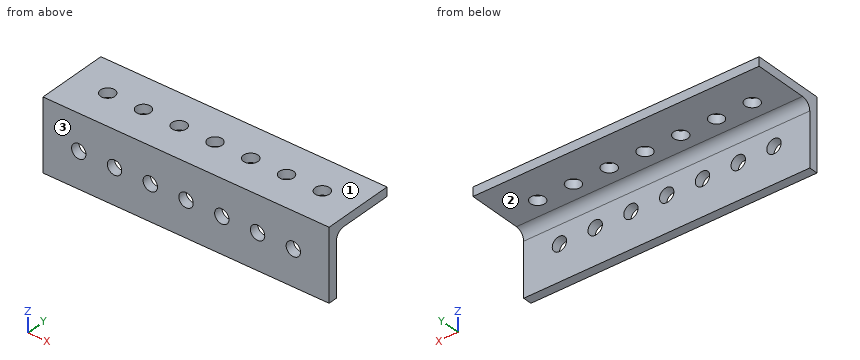
Autodesk Inventor part; units mm, degrees
ref_plane "YZ Plane" through (0, 0, 0) normal (1, 0, 0) x (0, 1, 0)
ref_plane "XZ Plane" through (0, 0, 0) normal (0, 1, 0) x (-1, 0, 0)
ref_plane "XY Plane" through (0, 0, 0) normal (0, 0, 1) x (1, 0, 0)
sketch "Sketch1" plane through (0, 0, 0) normal (1, 0, 0) x (0, 1, 0)
  line L0 (25.4, 0) -> (0, 0)
  line L1 (0, 0) -> (0, -25.4)
  line L2 (0, -25.4) -> (3.175, -25.4)
  line L3 (3.175, -25.4) -> (3.175, -3.175)
  line L4 (3.175, -3.175) -> (25.4, -3.175)
  line L5 (25.4, -3.175) -> (25.4, 0)
  dimension "d0" = 25.4
  dimension "d1" = 25.4
  dimension "d2" = 3.175
extrude "Extrusion1" add sketch "Sketch1" along normal mid plane 101.6
fillet "Fillet1" radius 3.175 1 edges at (0, 3.175, -3.175)
sketch "Sketch2" plane through (-50.8, 0, 0) normal (0, 0, 1) x (1, 0, 0)
  line L0 (0, 0) -> (0, 25.4)
  line L1 (101.6, 0) -> (0, 0)
  point P0 (50.8, 0)
  point P1 (12.7, 12.7)
  point P2 (0, 12.7)
  point P3 (25.4, 12.7)
  point P4 (38.1, 12.7)
  point P5 (50.8, 12.7)
  point P6 (63.5, 12.7)
  point P7 (76.2, 12.7)
  point P8 (88.9, 12.7)
  dimension "d6" = 12.7
  dimension "d9" = 12.7
hole "Hole1" at (-38.1, 12.7, 0) at (-25.4, 12.7, 0) at (-12.7, 12.7, 0) at (0, 12.7, 0) at (12.7, 12.7, 0) at (25.4, 12.7, 0) at (38.1, 12.7, 0) direction (0, 0, -1) diameter 5.1054 end through all
sketch "Sketch3" plane through (-50.8, 0, -25.4) normal (0, -1, 0) x (1, 0, 0)
  line L0 (0, 0) -> (0, 25.4)
  line L1 (101.6, 25.4) -> (0, 25.4)
  point P0 (50.8, 25.4)
  point P1 (12.7, 12.7)
  point P2 (0, 12.7)
  point P3 (25.4, 12.7)
  point P4 (38.1, 12.7)
  point P5 (50.8, 12.7)
  point P6 (63.5, 12.7)
  point P7 (76.2, 12.7)
  point P8 (88.9, 12.7)
  dimension "d21" = 12.7
  dimension "d24" = 12.7
hole "Hole2" at (-38.1, 0, -12.7) at (-25.4, 0, -12.7) at (-12.7, 0, -12.7) at (0, 0, -12.7) at (12.7, 0, -12.7) at (25.4, 0, -12.7) at (38.1, 0, -12.7) direction (0, 1, 0) diameter 5.1054 end through all
equation "\"d1\" = d0"
properties part number "GI - 008" material "Aluminum 6061"
Geometry: final body of the model. Coordinates: model frame, mm. Face numbers are marked on the shaded views. Give positions to 0.01 mm unless a question says otherwise; leave off trailing zeros. Order: outer loops, then holes, each group sorted by start corner. A loop starts at its lowest first (then second) coordinate and runs counter-clockwise, first axis right, second up. Notation, with made-up numbers: (18.25, -37) -> (32.25, -37) arc R18 ccw to (32.25, -18) -> close; hole circle Ø6 at (36.25, -31.75). An arc over 180 degrees is marked (long way). Write each question's results on one line, items separated by ' | '. Start each with the question number.
1) First-contact query: pin 1 (4.5 mm diameter, centred on x = 38.1, z = -12.7, fed in from +Y); pin 2 (15 mm diameter, centred on x = -9, y = 17, fed in from -Z) (3 decimals); pin 3 (6.5 mm diameter, centred on x = -25.4, z = -12.7, fed in from +Y) (3 decimals). Flat tips, straight axial feed; report the tip coordinate or a pass-through.
2) Section D-D (y = 18). Return loops of the section in (x, z) (3 decimals).
3) Line query: line 1 (Z direction, x = 38.1, y = 1.8); line 2 (Y direction, x = -32, z = -14.25) (3 decimals); line 3 (Y direction, x = -25.4, z = -1.55). Output: solid intervals per line, ascending. Write a range as from..to.
4) Section A-A (y = 12.7). Count the separate pieces of the cut face and the enclosed holes in it, then the cut area to 3 significant figures.
5) Section B-B (x = -38.1). Return loops of the section in (y, z) (3 decimals), then the cut area to 3 significant figures.
6) Draft query along Z for the marked faces 1, 2 and 3. Return one class per face: pulls with the +Z half, pulls with the -Z half, needs draft (parallel to the pull), parting line crosses it, or undercut.
Calculated:
1) pin 1: through | pin 2: z = -3.175 | pin 3: y = 3.175
2) outline: (-50.8, -3.175) -> (50.8, -3.175) -> (50.8, 0) -> (-50.8, 0) -> close
3) line 1: -25.4..-15.25, -10.15..0 | line 2: 0..3.175 | line 3: 0..10.15, 15.25..25.4
4) separate pieces: 8 | enclosed holes: 0 | area: 209 mm2
5) outline: (0, -25.4) -> (3.175, -25.4) -> (3.175, -15.253) -> (0, -15.253) -> close; (0, -10.147) -> (3.175, -10.147) -> (3.175, -6.35) arc R3.175 cw to (6.35, -3.175) -> (10.147, -3.175) -> (10.147, 0) -> (0, 0) -> close; (15.253, -3.175) -> (25.4, -3.175) -> (25.4, 0) -> (15.253, 0) -> close | area: 121 mm2
6) face 1: pulls with the +Z half | face 2: pulls with the -Z half | face 3: needs draft
